Design review of the part built by this model. Coordinates are the model's own, in mm. A direction names the side the tool comes from. Give positions to 0.01 mm unless a question says otherwise; leave off trailing zeros. Order: outer loops, then holes, each group sorted by start corner. A loop starts at its lowest first (then second) coordinate and runs counter-clockwise, first axis right, second up. Notation, with made-up numbers: (34, -20) -> (64, -20) arc R25 ccw to (64, -5) -> close; hole circle Ø9 at (67.5, -2.5). An arc over 180 degrees is marked (long way). Use a Markdown table: item, result. Add a question column.
```python
from build123d import *

# Parameters (mm, degrees)
BOSS_EXTRUDE1_DEPTH     = 10
SKETCH2_R               = 1.65
CUT_EXTRUDE1_DEPTH      = 26.395491135
BOSS_EXTRUDE2_START     = -10
BOSS_EXTRUDE2_DEPTH     = 10
CUT_EXTRUDE3_DEPTH      = 10
CUT_EXTRUDE3_DEPTH_BACK = 10
SKETCH8_R               = 1.4
SKETCH9_R               = 1.65
CUT_EXTRUDE4_DEPTH      = 46.090984648


with BuildPart() as part:
    # Sketch1 → Boss-Extrude1 (new body)
    with BuildSketch(Plane.XY):
        with BuildLine():
            Line((11.679694055, 24.106798453), (-3.320305945, 24.106798453))
            Line((-3.320305945, 24.106798453), (-3.320305945, 27.106798453))
            Line((-3.320305945, 27.106798453), (11.679694055, 27.106798453))
            ThreePointArc((11.679694055, 27.106798453), (18.679694055, 20.106798453), (11.679694055, 13.106798453))
            Line((11.679694055, 13.106798453), (-3.320305945, 13.106798453))
            Line((-3.320305945, 13.106798453), (-3.320305945, 16.606798453))
            Line((-3.320305945, 16.606798453), (9.743202382, 16.606798453))
            ThreePointArc((9.743202382, 16.606798453), (15.552677401, 19.106798453), (11.679694055, 24.106798453))
        make_face()
    extrude(amount=BOSS_EXTRUDE1_DEPTH)

    # Sketch2 → Cut-Extrude1 (cut, through all)
    with BuildSketch(Plane(origin=(0, 27.106798453, 0), x_dir=(1, 0, 0), z_dir=(0, 1, 0))):
        with Locations(Location((0.679694055, -5, 0), (0, 0, 180))):
            Circle(SKETCH2_R)
    extrude(amount=-CUT_EXTRUDE1_DEPTH, mode=Mode.SUBTRACT)

    # Sketch5 → Boss-Extrude2 (add)
    with BuildSketch(Plane.XY.offset(10).offset(BOSS_EXTRUDE2_START)):
        with BuildLine():
            Line((41.679694055, 17.106798453), (14.325445366, 17.106798453))
            ThreePointArc((14.325445366, 17.106798453), (12.113586102, 16.130400875), (9.743202382, 16.606798453))
            Line((9.743202382, 16.606798453), (-3.320305945, 16.606798453))
            Line((-3.320305945, 16.606798453), (-3.320305945, 13.106798453))
            Line((-3.320305945, 13.106798453), (41.679694055, 13.106798453))
            Line((41.679694055, 13.106798453), (41.679694055, 17.106798453))
        make_face()
    extrude(amount=BOSS_EXTRUDE2_DEPTH)

    # Sketch8 → Cut-Extrude3 (cut, two sides: drawn at the far end of the back side and taken through both)
    with BuildSketch(Plane(origin=(0, 13.948922433, 0), x_dir=(1, 0, 0), z_dir=(0, 1, 0)).offset(-CUT_EXTRUDE3_DEPTH_BACK)):
        with Locations((28.679694055, -5)):
            Circle(SKETCH8_R)
        with Locations((38.679694055, -5)):
            Circle(SKETCH8_R)
        with Locations((23.679694055, -5)):
            Circle(SKETCH8_R)
        with Locations((33.679694055, -5)):
            Circle(SKETCH8_R)
    extrude(amount=CUT_EXTRUDE3_DEPTH + CUT_EXTRUDE3_DEPTH_BACK, mode=Mode.SUBTRACT)

    # Sketch9 → Cut-Extrude4 (cut, through all)
    with BuildSketch(Plane(origin=(0, 27.106798453, 0), x_dir=(1, 0, 0), z_dir=(0, 1, 0))):
        with Locations(Location((0.679694055, -5, 0), (0, 0, 180))):
            Circle(SKETCH9_R)
    extrude(amount=-CUT_EXTRUDE4_DEPTH, mode=Mode.SUBTRACT)


solid = part.part
```
1) Add section D-D (z = 2). Give the boundary of the cut face in (x, y).
2) Insertion check: pin 1 (4 mm diameter, centred on x = 0.68, z = 5, fed in from -Y); pin 2 (5 mm diameter, centred on x = 35, z = 7.5, fed in from +Y); pin 3 (1 mm diameter, centred on y = 19, z = 5.5, fed in from -X); pin 4 (1 mm diameter, centred on y = 20, z = 3, fed in from -X). Each pin has a flat end and moves straight along its axis. Give the tip position at first contact, or say it passes through.
3) Add section A-A (z = 5). Give the number of separate pieces and of enclosed holes in the cut face, then the cut area to 3 significant figures.
4) Add section B-B (y = 14.75). Give the boundary of the cut face in (x, z).
5) The part is to be moulded in two halves that separate along X. For faces 3 (the cylindrical face through (22.28, 15.08, 4.94)), 4 (the cylindrical face through (15.526, 19.008, 4.93)), 5 (the flat face through (3, 16.607, 5)), 6 (the flat face through (-3.32, 15, 5)), say which applies: +X half, -X half, draft (parallel to the pull), parting line (faces both ways), or undercut.
6) Add section C-C (x = 7.5). Give the boundary of the cut face in (y, z), then the cut area to 3 significant figures.
7) Machinability: for faces 1 (the flat face through (4, 24.107, 5)), 2 (the flat face through (-3.32, 26, 5)), which of the approach directions +Z, -Z, +X, -X, +Y, -Y give a long, thin tool a straight path to every point of the face, cutting with its end or side? Answer none if there is none.
8) For L1, parallel to X at y = 15.5, z = 4.25; L2, parallel to Y at x = 6, z = 4.75; L3, parallel to Y at x = 23, z = 9.75, list the stretches that pass through material, from the lowest coordinate up. Write a range as [from, to].
Worked answers:
| question | item | result |
|---|---|---|
| 1 | outline | (-3.32, 13.11) -> (41.68, 13.11) -> (41.68, 17.11) -> (18, 17.11) arc R7 ccw to (11.68, 27.11) -> (-3.32, 27.11) -> (-3.32, 24.11) -> (11.68, 24.11) arc R4 cw (long way) to (9.74, 16.61) -> (-3.32, 16.61) -> close |
| 2 | pin 1 | y = 13.11 |
| 2 | pin 2 | y = 17.11 |
| 2 | pin 3 | x = 15.34 |
| 2 | pin 4 | x = 15.63 |
| 3 | separate pieces | 7 |
| 3 | enclosed holes | 0 |
| 3 | area | 184 mm^2 |
| 4 | outline | (-3.32, 0) -> (41.68, 0) -> (41.68, 10) -> (-3.32, 10) -> close; hole circle Ø3.3 at (0.68, 5); hole circle Ø2.8 at (23.68, 5); hole circle Ø2.8 at (28.68, 5); hole circle Ø2.8 at (33.68, 5); hole circle Ø2.8 at (38.68, 5) |
| 5 | face 3 | undercut |
| 5 | face 4 | undercut |
| 5 | face 5 | draft |
| 5 | face 6 | -X half |
| 6 | outline | (13.11, 0) -> (16.61, 0) -> (16.61, 10) -> (13.11, 10) -> close; (24.11, 0) -> (27.11, 0) -> (27.11, 10) -> (24.11, 10) -> close |
| 6 | area | 65.0 mm^2 |
| 7 | face 1 | +Z, -Z, -X |
| 7 | face 2 | +Z, -Z, -X, +Y, -Y |
| 8 | L1 | [-3.32, -0.79], [2.15, 22.5], [24.86, 27.5], [29.86, 32.5], [34.86, 37.5], [39.86, 41.68] |
| 8 | L2 | [13.11, 16.61], [24.11, 27.11] |
| 8 | L3 | [13.11, 17.11] |
